Could you check a few things on this model? Use its own coordinates, in mm. A direction names the side the tool comes from. Round coordinates to 2 decimals unless told otherwise and drop trailing zeros. Loops run counter-clockwise (first coordinate to the right, second up) from the corner with the lowest first, then second, coordinate; pieces in that order, holes last. Notation, with made-up numbers: M 38,20.5 L 55,20.5 A33 ccw 55,55.5 Z; hole C -24,-36 d10. An arc over 180 degrees is marked long. One line per item, written item: value. Start each with the question number.
Q1. Imagine slicing it at B-B (y = 15.5). Please give me the cut outline in (x, z), then the cut area to 3 significant figures.
Q2. Imagine slicing it at A-A (y = 84.5). Please give me the cut outline in (x, z), then the cut area to 3 significant figures.
Q3. Which directions (+Z, -Z, +X, -X, +Y, -Y) give clear straight access to the entire face, cutting with the end or side of a thin tool? Please do faces 1 (the face through (0, -53.767, 0)), 2 (the face through (22, 6.558, 7)), 3 (the face through (15.12, -29.62, 11.59)).
Q4. Thinking about a two-plate mould opening in Z: for faces 4 (the face through (-22, -2.967, 7)), 5 (the face through (5.705, 80.649, 0.749)), 6 (the face through (15.12, 53.2, 11.59)), which applies, released by +Z, released by -Z, zero draft, split by the parting line, or undercut?
Q5. Please list where these lines run through material, in increasing order: line 1 along Z through (x, y) = (0, 86); line 2 along Y through (x, z) = (18.5, 25.5).
Q6. Imagine slicing it at C-C (y = -0.5). Please give me the cut outline in (x, z), then the cut area to 3 significant figures.
Q7. I'm going to push flat-ended pins straight in: pin 1 Ø2 at (x, y) = (8, -10.5) entering from +Z; pin 2 Ø8 at (y, z) = (80, 11.5) entering from +X; pin 3 Ø1 at (y, z) = (44.5, 15.5) entering from -X. Where does each tip first touch, or does it pass through?
from build123d import *

# Parameters (mm, degrees)
F_1_2_20_TAPPED_HOLE1_D     = 11.50874
F_1_2_20_TAPPED_HOLE1_DEPTH = 29.21
F_1_2_20_TAPPED_HOLE1_TIP   = 3.45757432
FILLET1_R                   = 3.175


with BuildPart() as part:
    # Sketch1 → Revolve2 (revolve)
    with BuildSketch(Plane.XY):
        Polygon((-31.75, -2.966632853), (-31.75, 6.558367147), (-19.05, 6.558367147), (-19.05, 95.458367147), (0, 95.458367147), (0, 0), (0, -53.766632853), (-19.05, -53.766632853), (-19.05, -2.966632853), align=None)
    revolve(axis=Axis((0, 95.458367147, 0), (0, -1, 0)))

    # 1/2-20 Tapped Hole1
    with Locations(Plane.ZX.offset(95.458367147)):
        with Locations((0, 0)):
            Hole(F_1_2_20_TAPPED_HOLE1_D / 2, depth=F_1_2_20_TAPPED_HOLE1_DEPTH)
            with Locations((0, 0, -(F_1_2_20_TAPPED_HOLE1_DEPTH + F_1_2_20_TAPPED_HOLE1_TIP / 2))):  # 118° drill point
                Cone(0, F_1_2_20_TAPPED_HOLE1_D / 2, F_1_2_20_TAPPED_HOLE1_TIP, mode=Mode.SUBTRACT)

    # Fillet1
    fillet1_edges = [part.edges().sort_by_distance(p)[0] for p in [
        (19.05, 6.558367147, 0),
        (19.05, -2.966632853, 0),
    ]]
    fillet(fillet1_edges, radius=FILLET1_R)


solid = part.part
Report:
1. outline: C 0,0 d38.1
1. area: 1,140 mm²
2. outline: C 0,0 d38.1; hole C 0,0 d11.51
2. area: 1,040 mm²
3. face 1: +Z, -Z, +X, -X, -Y
3. face 2: +Y
3. face 3: -Y
4. face 4: zero draft
4. face 5: undercut
4. face 6: split by the parting line
5. line 1: z = -19.05 to -5.75, 5.75 to 19.05
5. line 2: y = -2.97 to 6.56
6. outline: C 0,0 d63.5
6. area: 3,170 mm²
7. pin 1: stops at z = 17.72
7. pin 2: stops at x = 17.51
7. pin 3: stops at x = -11.74
